```python
from build123d import *

# Parameters (mm, degrees)
F0_R     = 20
F1_DEPTH = 60
F2_R     = 20
F2_R_2   = 15
F3_DEPTH = 40
F5_DEPTH = 20
F6_R     = 1.5
F8_R     = 5
F9_DEPTH = 60


with BuildPart() as f1:
    # F0 (on Right) → F1 (new body)
    with BuildSketch(Plane.YZ):
        Circle(F0_R)
    extrude(amount=F1_DEPTH)

    # F2 (on face) → F3 (cut)
    with BuildSketch(Plane.YZ.offset(60)):
        Circle(F2_R)
        Circle(F2_R_2, mode=Mode.SUBTRACT)
    extrude(amount=-F3_DEPTH, mode=Mode.SUBTRACT)

    # F4 (on face) → F5 (cut)
    with BuildSketch(Plane.YZ.offset(20)):
        with BuildLine():
            Line((-18, -8.717798), (-18, 8.717798))
            ThreePointArc((-18, 8.717798), (-20, 0), (-18, -8.717798))
        make_face()
        with BuildLine():
            ThreePointArc((18, -8.717798), (20, 0), (18, 8.717798))
            Line((18, 8.717798), (18, -8.717798))
        make_face()
    extrude(amount=-F5_DEPTH, mode=Mode.SUBTRACT)

    # F6 (on Front) → F7 (revolve, cut)
    with BuildSketch(Plane.XZ):
        with Locations((50, 15)):
            Circle(F6_R)
    revolve(axis=Axis((60, 0, 0), (1, 0, 0)), mode=Mode.SUBTRACT)

    # F8 (on face) → F9 (cut)
    with BuildSketch(Plane.YZ.offset(60)):
        Circle(F8_R)
    extrude(amount=-F9_DEPTH, mode=Mode.SUBTRACT)


solid = f1.part
```
The listing builds one solid part. Answer for the finished solid, in the listing's coordinates (mm). A direction names the side the tool comes from. Give positions to 0.01 mm unless a question says otherwise; leave off trailing zeros. Write each loop counter-clockwise with the first axis right and the second up, starting at its lowest first coordinate (ties: lowest second). Pieces come first, ordered by that corner, then holes. Notation, with made-up numbers: (85, -17.5) - (111, -17.5) arc R27 cw to (111, 15.5) - close; hole circle Ø1 at (-13.5, -7). An arc over 180 degrees is marked (long way). Use one line per item in the form item = value. Start each with the question number.
1) Consider line 1 along Z through (x, y) = (30, 0); line 2 along Z through (x, y) = (18, 0); line 3 along X through (y, z) = (14, 9). Determine where each line is inside the solid, lowest interval first. Write a range as from..to.
2) Find section C-C on x = 4.5. Determine the outline of the cut face in (y, z).
3) The mould has two halves that part along Z. Classify faces 1 (the face through (55.81, -3.252, -14.643)), 2 (the face through (30.42, -1.08, -4.88)), 3 (the face through (20, -4, -15)), 4 (the face through (10, 0, 20)): pulls with the +Z half, pulls with the -Z half, needs draft (parallel to the pull), parting line crosses it, or undercut.
4) Flat-ended cylindrical pins translate along their axes: pin 1 Ø12 at (x, z) = (38, 1) entering from -Y; pin 2 Ø10 at (x, y) = (33.5, -7) entering from -Z; pin 3 Ø2 at (x, y) = (13.5, -13.5) entering from -Z; pin 4 Ø1 at (y, z) = (-2, 2) entering from +X. Find the tip coordinate at first contact, or state that the pin passes through.
5) Find section A-A on y = 0. Determine the outline of the cut face in (x, z), plus the area to 3 significant figures.
6) Find section D-D on x = 22.5. Determine the outline of the cut face in (y, z).
7) A tool of negligible diameter and unlimited length cuts with its end or side. For faces 5 (the face through (10, -18, 0)), 6 (the face through (34.45, -14.985, 0.66)), from which of +Z, -Z, +X, -X, +Y, -Y can it reach the whole face along a straight path? Write none if from no direction.
8) Find section B-B on z = 0. Determine the outline of the cut face in (x, y).
Geometry results:
q1.line_1 = -15..-5, 5..15
q1.line_2 = -20..-5, 5..20
q1.line_3 = 0..20
q2.outline = (-18, -8.72) arc R20 ccw to (18, -8.72) - (18, 8.72) arc R20 ccw to (-18, 8.72) - close; hole circle Ø10 at (0, 0)
q3.face_1 = parting line crosses it
q3.face_2 = undercut
q3.face_3 = needs draft
q3.face_4 = pulls with the +Z half
q4.pin_1 = -15
q4.pin_2 = -14.87
q4.pin_3 = -15.61
q4.pin_4 = through
q5.outline = (0, -20) - (20, -20) - (20, -15) - (48.5, -15) arc R1.5 cw to (51.5, -15) - (60, -15) - (60, -5) - (0, -5) - close; (0, 5) - (60, 5) - (60, 15) - (51.5, 15) arc R1.5 cw to (48.5, 15) - (20, 15) - (20, 20) - (0, 20) - close
q5.area = 1,390 mm2
q6.outline = circle Ø30 at (0, 0); hole circle Ø10 at (0, 0)
q7.face_5 = +Z, -Z, +X, -X, -Y
q7.face_6 = +X
q8.outline = (0, -18) - (20, -18) - (20, -15) - (48.5, -15) arc R1.5 cw to (51.5, -15) - (60, -15) - (60, -5) - (0, -5) - close; (0, 5) - (60, 5) - (60, 15) - (51.5, 15) arc R1.5 cw to (48.5, 15) - (20, 15) - (20, 18) - (0, 18) - close
